Autodesk Inventor part; units mm, degrees
ref_plane "YZ Plane" through (0, 0, 0) normal (1, 0, 0) x (0, 1, 0)
ref_plane "XZ Plane" through (0, 0, 0) normal (0, 1, 0) x (-1, 0, 0)
ref_plane "XY Plane" through (0, 0, 0) normal (0, 0, 1) x (1, 0, 0)
sketch "Sketch1" plane through (0, 0, 0) normal (0, 1, 0) x (-1, 0, 0)
  circle A0 centre (0, 0) radius 36.5125
  circle A1 centre (0, 0) radius 39.6875
  dimension "d0" = 73.025
  dimension "d1" = 79.375
extrude "Extrusion1" add sketch "Sketch1" along normal mid plane 1219.2
sketch "Sketch2" plane through (0, 0, 0) normal (1, 0, 0) x (0, 1, 0)
  line L0 (-609.6, 4.7625) -> (-431.8, 4.7625)
  line L1 (-431.8, 4.7625) -> (-431.8, -4.7625)
  line L2 (-431.8, -4.7625) -> (-609.6, -4.7625)
  line L3 (-609.6, -4.7625) -> (-609.6, 4.7625)
  line L4 (-609.6, 39.6875) -> (-609.6, -39.6875)
  line L5 (-609.6, 39.6875) -> (-609.6, -39.6875)
  line L6 (609.6, -39.6875) -> (609.6, 39.6875)
  line L7 (-609.6, -39.6875) -> (609.6, -39.6875)
  line L8 (-419.1, 4.7625) -> (-241.3, 4.7625)
  line L9 (-241.3, 4.7625) -> (-241.3, -4.7625)
  line L10 (-241.3, -4.7625) -> (-419.1, -4.7625)
  line L11 (-419.1, -4.7625) -> (-419.1, 4.7625)
  point P0 (0, 0)
  dimension "d4" = 177.8
  dimension "d5" = 9.525
  dimension "d6" = 34.925
  dimension "d12" = 177.8
  dimension "d13" = 9.525
  dimension "d14" = 12.7
extrude "Extrusion2" cut sketch "Sketch2" along normal blind 76.2
pattern_circular "Circular Pattern1" count 3 over 360 about axis through (0, 0, 0) along (0, 1, 0) of "Extrusion2"
equation "\"d13\" = d5"
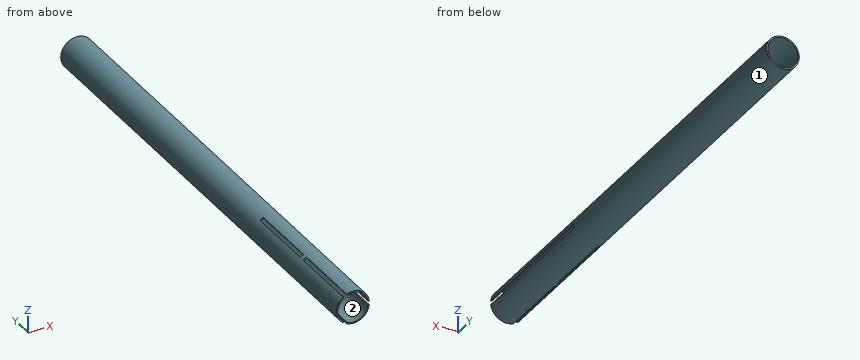
Read the model definition and answer for the solid it produces. Units are mm, in the model's axes. Face numbers are marked on the shaded views. Round coordinates to 2 decimals unless told otherwise and drop trailing zeros. Order: outer loops, then holes, each group sorted by start corner. A loop starts at its lowest first (then second) coordinate and runs counter-clockwise, first axis right, second up. Notation, with made-up numbers: (52, 42.25) - (104, 42.25) arc R25 ccw to (104, 61.25) - close; hole circle Ø3 at (-2.5, 24). An arc over 180 degrees is marked (long way). Use one line per item in the form item = value. Start each with the question number.
(1) Find the intervals of material crossed by line 1 along Z through (x, y) = (0, -50); line 2 along X through (y, z) = (3.5, 2), in increasing order. Write a range as from..to.
(2) The part is cut by section B-B (x = 0). Give the vertices of the cut face in (y, z).
(3) The part is cut by section C-C (z = -15). Give the vertices of the cut face in (x, y).
(4) The part is cut by section A-A (y = -494). Give the vertices of the cut face in (x, z) (1 decimal), then the cut area to 3 significant figures.
(5) Flat-ended cylindrical pins translate along their axes: pin 1 Ø8 at (y, z) = (355.5, -20.5) entering from +X (3 decimals); pin 2 Ø4 at (y, z) = (-11, 27.5) entering from -X; pin 3 Ø2.5 at (x, z) = (-19.5, -32.5) entering from -Y; pin 4 Ø6 at (x, z) = (-17, 31) entering from +Y. Find the tip coordinate at first contact, or state that the pin passes through.
(6) Determine the mould class of the marked faces 1 and 2 for opening direction Z: +Z half, -Z half, draft (parallel to the pull), parting line (faces both ways), or undercut.
(7) The part is cut by section D-D (y = -1.5). Give the vertices of the cut face in (x, z) (1 decimal).
Checked values:
q1.line_1 = -39.69..-36.51, 36.51..39.69
q1.line_2 = -39.64..-36.46, 36.46..39.64
q2.outline = (-609.6, -39.69) - (609.6, -39.69) - (609.6, -36.51) - (-609.6, -36.51) - close; (-609.6, 36.51) - (609.6, 36.51) - (609.6, 39.69) - (-609.6, 39.69) - close
q3.outline = (-36.74, -609.6) - (-33.29, -609.6) - (-33.29, 609.6) - (-36.74, 609.6) - close; (33.29, -609.6) - (36.74, -609.6) - (36.74, 609.6) - (33.29, 609.6) - close
q4.outline = (-23.8, -31.7) - (-22.2, -29) arc R36.5 cw to (-22.2, 29) - (-23.8, 31.7) arc R39.7 ccw to start; (-15.6, -36.5) arc R39.7 ccw to (39.4, -4.8) - (36.2, -4.8) arc R36.5 cw to (-14, -33.7) - close; (-15.6, 36.5) - (-14, 33.7) arc R36.5 cw to (36.2, 4.8) - (39.4, 4.8) arc R39.7 ccw to start
q4.area = 669 mm^2
q5.pin_1 = 36.095
q5.pin_2 = -30.41
q5.pin_3 = -431.8
q5.pin_4 = 609.6
q6.face_1 = parting line
q6.face_2 = undercut
q7.outline = circle Ø79.4 at (0, 0); hole circle Ø73 at (0, 0)
